Autodesk Inventor part; units mm, degrees
ref_plane "YZ Plane" through (0, 0, 0) normal (1, 0, 0) x (0, 1, 0)
ref_plane "XZ Plane" through (0, 0, 0) normal (0, 1, 0) x (-1, 0, 0)
ref_plane "XY Plane" through (0, 0, 0) normal (0, 0, 1) x (1, 0, 0)
sketch "Sketch1" plane through (0, 0, 0) normal (0, 0, 1) x (1, 0, 0)
  line L0 (80, 30) -> (-80, 30)
  line L1 (-80, 30) -> (-80, -30)
  line L2 (-80, -30) -> (80, -30)
  line L3 (80, -30) -> (80, 30)
  line L4 (80, 30) -> (-80, -30) construction
  line L5 (-80, 30) -> (80, -30) construction
  line L6 (-20, -30) -> (-80, -30)
  line L7 (-80, -30) -> (-80, 30)
  line L8 (-80, 30) -> (-20, 30)
  line L9 (-20, 30) -> (-20, -30)
  line L10 (-20, -30) -> (-80, 30) construction
  line L11 (-80, -30) -> (-20, 30) construction
  line L12 (20, -30) -> (80, -30)
  line L13 (80, -30) -> (80, 30)
  line L14 (80, 30) -> (20, 30)
  line L15 (20, 30) -> (20, -30)
  line L16 (20, -30) -> (80, 30) construction
  line L17 (80, -30) -> (20, 30) construction
  line L18 (0, 30) -> (0, -30) construction
  point P0 (0, 0)
  point P1 (-50, 0)
  point P2 (50, 0)
  point P3 (20, 30)
  point P4 (20, -30)
  point P5 (-20, -30)
  point P6 (-20, 30)
  dimension "d0" = 160
  dimension "d1" = 60
  dimension "d2" = 40
extrude "Extrusion1" add sketch "Sketch1" along normal blind 10 contours L3 L2 L15 L0 | L9 L2 L1 L0
sketch "Sketch2" plane through (0, 0, 10) normal (0, 0, 1) x (1, 0, 0)
  line L0 (-80, -30) -> (-20, -30)
  line L1 (80, -24) -> (-80, -24)
  line L2 (-80, -24) -> (-80, -30)
  line L3 (-80, -30) -> (80, -30)
  line L4 (80, -30) -> (80, -24)
  line L5 (80, -24) -> (-80, -30) construction
  line L6 (-80, -24) -> (80, -30) construction
  line L7 (80, -30) -> (80, 30)
  point P0 (0, 0)
  point P1 (0, -27)
  dimension "d5" = 6
extrude "Extrusion2" add sketch "Sketch2" along normal blind 110
sketch "Sketch3" plane through (0, 0, 0) normal (0, 0, -1) x (-1, 0, 0)
  line L0 (53, 7.5) -> (43, 7.5)
  line L1 (43, 7.5) -> (43, -7.5)
  line L2 (43, -7.5) -> (53, -7.5)
  line L3 (53, -7.5) -> (53, 7.5)
  line L4 (53, 7.5) -> (43, -7.5) construction
  line L5 (43, 7.5) -> (53, -7.5) construction
  line L6 (-43, 7.5) -> (-53, 7.5)
  line L7 (-53, 7.5) -> (-53, -7.5)
  line L8 (-53, -7.5) -> (-43, -7.5)
  line L9 (-43, -7.5) -> (-43, 7.5)
  line L10 (-43, 7.5) -> (-53, -7.5) construction
  line L11 (-53, 7.5) -> (-43, -7.5) construction
  line L12 (80, -30) -> (-80, -30) construction
  line L13 (0, -30) -> (0, 0) construction
  point P0 (48, 0)
  point P1 (-48, 0)
  point P2 (48, 0)
  dimension "d8" = 10
  dimension "d9" = 15
  dimension "d10" = 48
extrude "Extrusion3" cut sketch "Sketch3" against normal through all
sketch "Sketch4" plane through (0, 0, 0) normal (0, 0, -1) x (-1, 0, 0)
  line L0 (-70, -20) -> (70, -20) construction
  line L1 (70, -20) -> (70, 20) construction
  line L2 (70, 20) -> (-70, 20) construction
  line L3 (-70, 20) -> (-70, -20) construction
  line L4 (-70, -20) -> (70, 20) construction
  line L5 (70, -20) -> (-70, 20) construction
  circle A0 centre (70, 20) radius 1.25
  circle A1 centre (-70, 20) radius 1.25
  circle A2 centre (-70, -20) radius 1.25
  circle A3 centre (70, -20) radius 1.25
  point P0 (0, 0)
  dimension "d13" = 140
  dimension "d14" = 40
  dimension "d16" = 2.5
extrude "Extrusion4" cut sketch "Sketch4" against normal through all
sketch "Sketch5" plane through (-20, -24, 10) normal (0, 1, 0) x (1, 0, 0)
  line L0 (59.5, -13) -> (-19.5, -13) construction
  line L1 (-19.5, -13) -> (-19.5, -113) construction
  line L2 (-19.5, -113) -> (59.5, -113) construction
  line L3 (59.5, -113) -> (59.5, -13) construction
  line L4 (59.5, -13) -> (-19.5, -113) construction
  line L5 (-19.5, -13) -> (59.5, -113) construction
  line L6 (100, -110) -> (-60, -110) construction
  line L7 (55.5, -17) -> (-2.5, -17) construction
  line L8 (-2.5, -17) -> (-2.5, -103) construction
  line L9 (-2.5, -103) -> (55.5, -103) construction
  line L10 (55.5, -103) -> (55.5, -17) construction
  line L11 (55.5, -17) -> (-2.5, -103) construction
  line L12 (-2.5, -17) -> (55.5, -103) construction
  circle A0 centre (-2.5, -17) radius 1.75
  circle A1 centre (55.5, -17) radius 1.75
  circle A2 centre (-2.5, -103) radius 1.75
  circle A3 centre (55.5, -103) radius 1.75
  point P0 (20, 10)
  point P1 (20, -63)
  point P2 (20, -63)
  point P3 (26.5, -60)
  point P4 (20, -63)
  point P5 (26.5, -60)
  dimension "d19" = 3
  dimension "d20" = 79
  dimension "d21" = 100
  dimension "d22" = 58
  dimension "d23" = 86
  dimension "d26" = 4
  dimension "d27" = 4
  dimension "d28" = 3.5
extrude "Extrusion5" cut sketch "Sketch5" against normal through all
properties part number "electrical_system_fix_board"
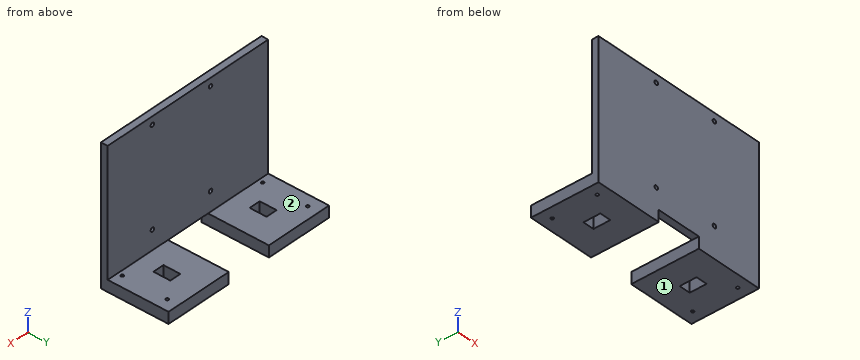
Input: part model. Units: mm. Frame: model coordinates. Face numbers are marked on the shaded views. A direction names the side the tool comes from. Give positions to 0.01 mm unless a question says otherwise; leave off trailing zeros. Order: outer loops, then holes, each group sorted by start corner. A loop starts at its lowest first (then second) coordinate and runs counter-clockwise, first axis right, second up. Notation, with made-up numbers: (56.5, 11) -> (95.5, 11) arc R25 ccw to (95.5, 23) -> close; hole circle Ø6 at (61.25, 23). An arc over 180 degrees is marked (long way). Use one line per item in the form item = value.
1) Section B-B, the plane y = 1. Return loops of the section in (x, z).
Response values:
outline = (-80, 0) -> (-53, 0) -> (-53, 10) -> (-80, 10) -> close; (-43, 0) -> (-20, 0) -> (-20, 10) -> (-43, 10) -> close; (20, 0) -> (43, 0) -> (43, 10) -> (20, 10) -> close; (53, 0) -> (80, 0) -> (80, 10) -> (53, 10) -> close
2) Line query: probe 1 along X at (y, z) = (-27.7, 27); probe 2 along Y at (x, z) = (70, 3); probe 3 along Z at (x, y) = (35, -25). Output: solid intervals per line, ascending.
Response values:
probe_1 = -80 to -24.25, -20.75 to 33.75, 37.25 to 80
probe_2 = -30 to -21.25, -18.75 to 18.75, 21.25 to 30
probe_3 = 0 to 25.32, 28.68 to 111.32, 114.68 to 120
3) Reachability of the marked faces 1 and 2 from +Z, -Z, +X, -X, +Y, -Y: full face, straight path, thin tool, end or side. Return the list, or none.
Response values:
face_1 = -Z, +X, -X, +Y, -Y
face_2 = +Z, +X, -X, +Y
4) Section D-D, the plane y = 17. Return loops of the section in (x, z).
Response values:
outline = (-80, 0) -> (-20, 0) -> (-20, 10) -> (-80, 10) -> close; (20, 0) -> (80, 0) -> (80, 10) -> (20, 10) -> close
5) Section A-A, the plane x = 45. Return loops of the section in (y, z), and give its area (3 significant figures).
Response values:
outline = (-30, 0) -> (-7.5, 0) -> (-7.5, 10) -> (-24, 10) -> (-24, 120) -> (-30, 120) -> close; (7.5, 0) -> (30, 0) -> (30, 10) -> (7.5, 10) -> close
area = 1,110 mm^2
6) First-contact query: pin 1 Ø3 at (x, z) = (35.5, 27) entering from +Y; pin 2 Ø1.8 at (x, y) = (-4, -26) entering from -Z; pin 3 Ø12 at (x, y) = (-27, 19) entering from +Z. Flat tips, straight axial feed; report the tip coordinate or a pass-through.
Response values:
pin_1 = through
pin_2 = 10
pin_3 = 10
7) Section C-C, the plane z = 113. Return loops of the section in (x, y).
Response values:
outline = (-80, -30) -> (-24.25, -30) -> (-24.25, -24) -> (-80, -24) -> close; (-20.75, -30) -> (33.75, -30) -> (33.75, -24) -> (-20.75, -24) -> close; (37.25, -30) -> (80, -30) -> (80, -24) -> (37.25, -24) -> close
